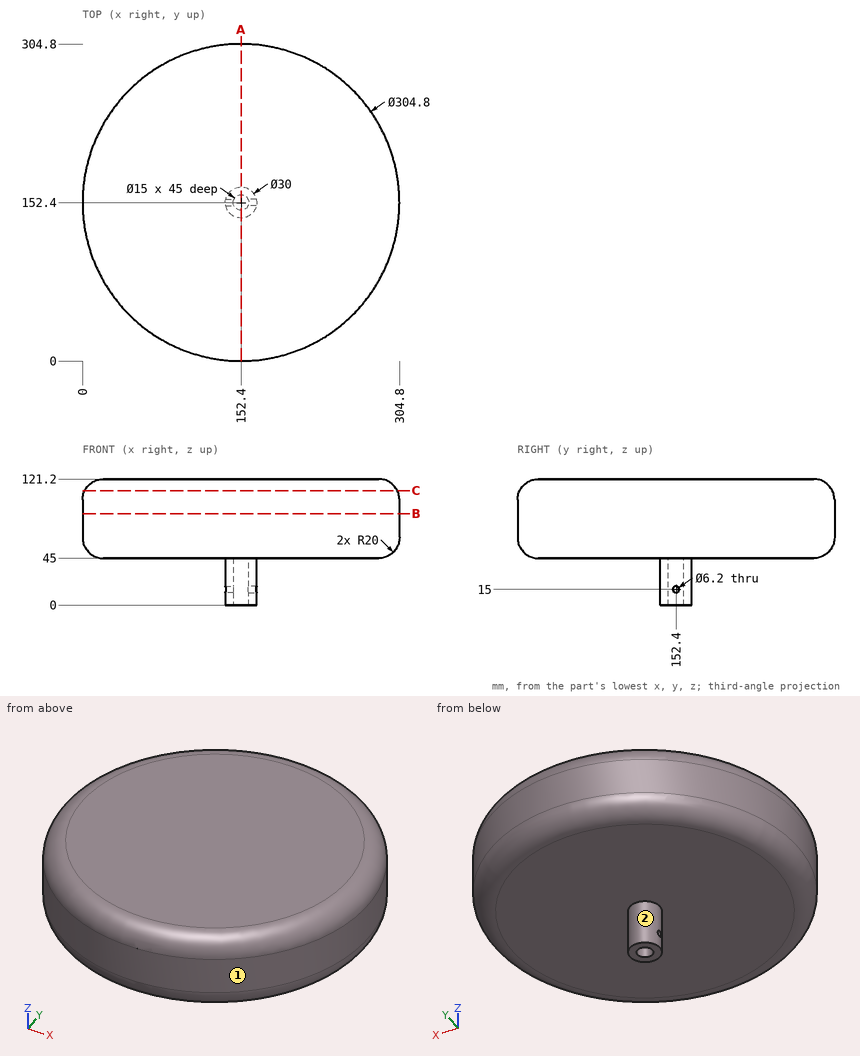
Part print with two shaded views. Sizes in mm from the minimum x, y, z corner. A direction names the side the tool comes from. Coordinates: 2 decimals unless noted, no trailing zeros. Write each loop counter-clockwise with the first axis right and the second up, starting at its lowest first coordinate (ties: lowest second). Pieces come first, ordered by that corner, then holes. Notation, with made-up numbers: (-36, 9) - (5, 9) arc R37 ccw to (5, 45) - close; hole circle Ø9 at (62, 16.25). An arc over 180 degrees is marked (long way). One line per item, written item: value. Start each with the question number.
1. Slice it at C-C (z = 110). Write the cut outline in (x, y), plus the area to 3 significant figures.
2. Probe line 1 (Z direction, x = 163, y = 152); line 2 (Y direction, x = 152.4, z = 18); line 3 (Z direction, x = 174, y = 109.5). List the from-to ranges inside material, lowest first. Write a range as from..to.
3. Flat gauge pins, fed straight in: pin 1 (10 mm diameter, centred on y = 152.4, z = 15, fed in from +X); pin 2 (5 mm diameter, centred on y = 222.5, z = 46.5, fed in from +X); pin 3 (12 mm diameter, centred on y = 189.5, z = 56.5, fed in from -X). Where does each tip first touch, or does it go through?
4. Tool access for the marked faces 1 and 2: list every direction of +Z, -Z, +X, -X, +Y, -Y with a clear straight run to the whole face (end or side of a thin tool).
5. Slice it at A-A (x = 152.4). Write the cut outline in (y, z), plus the area to 3 significant figures.
6. Slice it at B-B (z = 88). Write the cut outline in (x, y), plus the area to 3 significant figures.
Answers below:
1. outline: circle Ø300.72 at (152.4, 152.4)
1. area: 71,000 mm^2
2. line 1: z = 0..11.93, 18.07..121.2
2. line 2: y = 137.4..144.9, 159.9..167.4
2. line 3: z = 45..121.2
3. pin 1: stops at x = 167.4
3. pin 2: stops at x = 278.88
3. pin 3: stops at x = 4.05
4. face 1: +Z, -Z
4. face 2: -Z
5. outline: (0, 65) arc R20 ccw to (20, 45) - (137.4, 45) - (137.4, 0) - (144.9, 0) - (144.9, 45) - (159.9, 45) - (159.9, 0) - (167.4, 0) - (167.4, 45) - (284.8, 45) arc R20 ccw to (304.8, 65) - (304.8, 101.2) arc R20 ccw to (284.8, 121.2) - (20, 121.2) arc R20 ccw to (0, 101.2) - close
5. area: 23,600 mm^2
6. outline: circle Ø304.8 at (152.4, 152.4)
6. area: 73,000 mm^2
